For this review, take the finished solid that the model builds, in its own axes (mm). Coordinates: 2 decimals unless noted, no trailing zeros. Write each loop counter-clockwise with the first axis right and the second up, starting at its lowest first coordinate (ties: lowest second). Pieces come first, ordered by that corner, then holes. Notation, with made-up numbers: M 70.5,1 L 81.5,1 A13 cw 81.5,12 Z; hole C -32.75,26.25 d2. An arc over 180 degrees is marked long. Return JSON: item names as keys, results as strings.
```python
from build123d import *

# Parameters (mm, degrees)
EXTRUDE_1_DEPTH     = 3
SKETCH_2_R          = 1.55
CUT_EXTRUDE_1_DEPTH = 92.050809991
SKETCH_3_R          = 2.05
CUT_EXTRUDE_2_DEPTH = 92.050809991
SKETCH_4_W          = 3
SKETCH_4_H          = 40.476527492
CUT_EXTRUDE_3_DEPTH = 10
EXTRUDE_2_DEPTH     = 3
SKETCH_6_W          = 20
SKETCH_6_H          = 40
CUT_EXTRUDE_4_DEPTH = 4
FILLET_1_R          = 3
SKETCH_7_R          = 5
SKETCH_7_W          = 31
SKETCH_7_H          = 36
CUT_EXTRUDE_5_DEPTH = 4
SKETCH_8_R          = 2
CUT_EXTRUDE_6_DEPTH = 4
SKETCH_9_R          = 2
CUT_EXTRUDE_7_DEPTH = 4
FILLET_2_R          = 4


with BuildPart() as part:
    # 草图1 → 凸台-拉伸1 (new body)
    with BuildSketch(Plane.XY):
        Polygon((-32.5, 40), (-25, 40), (-10, 55), (-10, 85), (10, 85), (10, 55), (25, 40), (32.5, 40), (32.5, 0), (-32.5, 0), align=None)
    extrude(amount=EXTRUDE_1_DEPTH)

    # 草图2 → 切除-拉伸1 (cut, through all)
    with BuildSketch(Plane.XY.offset(3)):
        with Locations((-6, 81)):
            Circle(SKETCH_2_R)
        with Locations(Location((-6, 59, 0), (0, 0, 180))):
            Circle(SKETCH_2_R)
        with Locations((6, 59)):
            Circle(SKETCH_2_R)
        with Locations(Location((6, 81, 0), (0, 0, 180))):
            Circle(SKETCH_2_R)
    extrude(amount=-CUT_EXTRUDE_1_DEPTH, mode=Mode.SUBTRACT)

    # 草图3 → 切除-拉伸2 (cut, through all)
    with BuildSketch(Plane.XY.offset(3)):
        with Locations((-25, 26)):
            Circle(SKETCH_3_R)
        with Locations(Location((-25, 14, 0), (0, 0, 180))):
            Circle(SKETCH_3_R)
        with Locations((25, 14)):
            Circle(SKETCH_3_R)
        with Locations(Location((25, 26, 0), (0, 0, 180))):
            Circle(SKETCH_3_R)
    extrude(amount=-CUT_EXTRUDE_2_DEPTH, mode=Mode.SUBTRACT)

    # 草图4 → 切除-拉伸3 (cut)
    with BuildSketch(Plane.XY.offset(3)):
        with Locations((31, 19.761736254)):
            Rectangle(SKETCH_4_W, SKETCH_4_H)
        with Locations((-31, 19.761736254)):
            Rectangle(SKETCH_4_W, SKETCH_4_H)
    extrude(amount=-CUT_EXTRUDE_3_DEPTH, mode=Mode.SUBTRACT)

    # 草图5 → 凸台-拉伸2 (add)
    with BuildSketch(Plane.XY.offset(3)):
        Polygon((-125, 40), (-125, -84), (125, -84), (125, 40), (68, 40), (68, -10), (29.5, -10), (29.5, 0), (-29.5, 0), (-29.5, -10), (-68, -10), (-68, 40), align=None)
    extrude(amount=-EXTRUDE_2_DEPTH)

    # 草图6 → 切除-拉伸4 (cut)
    with BuildSketch(Plane.XY.offset(3)):
        with Locations((10, -64)):
            Rectangle(SKETCH_6_W, SKETCH_6_H)
        with Locations((-10, -64)):
            Rectangle(SKETCH_6_W, SKETCH_6_H)
    extrude(amount=-CUT_EXTRUDE_4_DEPTH, mode=Mode.SUBTRACT)

    # 圆角1
    fillet_1_edges = [part.edges().sort_by_distance(p)[0] for p in [
        (68, -10, 1.5),
        (68, 40, 1.5),
        (125, 40, 1.5),
        (125, -84, 1.5),
        (-125, -84, 1.5),
        (-125, 40, 1.5),
        (-68, 40, 1.5),
        (-68, -10, 1.5),
        (-29.5, -10, 1.5),
        (29.5, -10, 1.5),
        (20, -84, 1.5),
        (-20, -84, 1.5),
        (-20, -44, 1.5),
        (20, -44, 1.5),
        (-25, 40, 1.5),
        (-10, 55, 1.5),
        (-10, 85, 1.5),
        (10, 85, 1.5),
        (10, 55, 1.5),
        (25, 40, 1.5),
        (29.5, 40, 1.5),
        (-29.5, 40, 1.5),
    ]]
    fillet(fillet_1_edges, radius=FILLET_1_R)

    # 草图7 → 切除-拉伸5 (cut)
    with BuildSketch(Plane.XY.offset(3)):
        with Locations((72, -66)):
            Circle(SKETCH_7_R)
        with Locations((-72, -66)):
            Circle(SKETCH_7_R)
        with Locations((111.5, -20)):
            Rectangle(SKETCH_7_W, SKETCH_7_H)
        with Locations((-111.5, -20)):
            Rectangle(SKETCH_7_W, SKETCH_7_H)
    extrude(amount=-CUT_EXTRUDE_5_DEPTH, mode=Mode.SUBTRACT)

    # 草图8 → 切除-拉伸6 (cut)
    with BuildSketch(Plane.XY.offset(3)):
        with Locations((73, 26)):
            Circle(SKETCH_8_R)
        with Locations((73, 14)):
            Circle(SKETCH_8_R)
        with Locations((-73, 14)):
            Circle(SKETCH_8_R)
        with Locations((-73, 26)):
            Circle(SKETCH_8_R)
    extrude(amount=-CUT_EXTRUDE_6_DEPTH, mode=Mode.SUBTRACT)

    # 草图9 → 切除-拉伸7 (cut)
    with BuildSketch(Plane.XY.offset(3)):
        with Locations((110, -58)):
            Circle(SKETCH_9_R)
        with Locations((110, -70)):
            Circle(SKETCH_9_R)
        with Locations((-110, -70)):
            Circle(SKETCH_9_R)
        with Locations((-110, -58)):
            Circle(SKETCH_9_R)
    extrude(amount=-CUT_EXTRUDE_7_DEPTH, mode=Mode.SUBTRACT)

    # 圆角2
    fillet_2_edges = [part.edges().sort_by_distance(p)[0] for p in [
        (-125, -38, 1.5),
        (-125, -2, 1.5),
        (125, -38, 1.5),
        (125, -2, 1.5),
        (-96, -2, 1.5),
        (-96, -38, 1.5),
        (96, -38, 1.5),
        (96, -2, 1.5),
    ]]
    fillet(fillet_2_edges, radius=FILLET_2_R)


solid = part.part
```
1. We need section D-D (x = -45). State the section outline as (y, z) points, plus the area to 3 significant figures.
Checks:
{"outline": "M -84,0 L -10,0 L -10,3 L -84,3 Z", "area": "222 mm2"}
2. We need section B-B (z = 1.2). Give the number of separate pieces and of enclosed holes in the cut face, plus the area to 3 significant figures.
Checks:
{"separate pieces": "1", "enclosed holes": "18", "area": "24,200 mm2"}
3. We need section A-A (x = 104.5). State the section outline as (y, z) points, plus the area to 3 significant figures.
Checks:
{"outline": "M -84,0 L -38,0 L -38,3 L -84,3 Z; M -2,0 L 40,0 L 40,3 L -2,3 Z", "area": "264 mm2"}
4. Draft analysis for pull direction Y (two halves, no side actions). For faces 1 (the face through (-69, -62, 2)), 2 (the face through (-2, -17, 0)), 3 (the face through (-18, 47, 1)), 4 (the face through (75, -62, 2)), state which applies: +Y half, -Y half, draft (parallel to the pull), parting line (faces both ways), or undercut.
Checks:
{"face 1": "undercut", "face 2": "draft", "face 3": "+Y half", "face 4": "undercut"}
5. We need section C-C (y = 67). State the section outline as (x, z) points.
Checks:
{"outline": "M -10,0 L 10,0 L 10,3 L -10,3 Z"}
6. Clearance check with flat-ended pins moving along their axes: pin 1 Ø1.5 at (x, z) = (-114, 1.5) entering from +Y; pin 2 Ø0.9 at (x, z) = (-40.5, 1.5) entering from +Y. State where each tip first meets the part, or that it passes through.
Checks:
{"pin 1": "y = 40", "pin 2": "y = -10"}
7. Wall thickness on L1, parallel to X at y = 23, z = 1.55; L2, parallel to Y at x = -25, z = 2; L3, parallel to X at y = 81, z = 0.75: over which ranges is each line inside the solid? List them lowest first. Write a range as from..to.
Checks:
{"L1": "-125..-68, -29.5..29.5, 68..125", "L2": "-84..11.95, 16.05..23.95, 28.05..40.27", "L3": "-10..-7.55, -4.45..4.45, 7.55..10"}
